from build123d import *

# Parameters (mm, degrees)
F2_DEPTH = 7.62


with BuildPart() as f2:
    # F1 (on Right) → F2 (new body)
    with BuildSketch(Plane.YZ):
        Polygon((-9.930916, 15.784562), (-9.930916, -51.809832), (9.089336, -51.809832), (9.089336, 15.709758), align=None)
        Polygon((-9.930916, -51.809832), (-30.802712, -51.809832), (-30.802712, -67.667425), (48.981383, -67.146659), (48.981383, -51.809832), (9.089336, -51.809832), align=None)
    extrude(amount=-F2_DEPTH)


solid = f2.part
Check sheet for the modelled part. Datum: model origin and axes. Units: mm. A direction names the side the tool comes from. Give positions to 0.01 mm unless a question says otherwise; leave off trailing zeros. Write each loop counter-clockwise with the first axis right and the second up, starting at its lowest first coordinate (ties: lowest second). Pieces come first, ordered by that corner, then holes. Notation, with made-up numbers: (-21, 65) -> (33, 65) arc R20 cw to (33, 72) -> close; hole circle Ø4 at (40, -17.5). An arc over 180 degrees is marked (long way). One line per item, written item: value. Start each with the question number.
Item 1: Material ranges on probe 1 along Y at (x, z) = (-4, -24); probe 2 along Z at (x, y) = (-4.5, 45.5); probe 3 along Z at (x, y) = (-0.75, 8), recorded low to high. Write a range as from..to.
Item 2: Gauge pin test, flat ends, axial feed: pin 1 (3 mm diameter, centred on x = -5, y = 22, fed in from -Z); pin 2 (2.5 mm diameter, centred on x = -2.5, z = -26.5, fed in from -Y); pin 3 (2.5 mm diameter, centred on x = -4.5, y = -16.5, fed in from +Z). Record the tip position at first contact, or that the pin passes through.
Item 3: Tool access check on faces 1 (the flat face through (-4, 29, -51.81)), 2 (the flat face through (-4, -20, -51.81)), 3 (the flat face through (-4, 48.981, -60)). Record the directions out of +Z, -Z, +X, -X, +Y, -Y that give a thin tool (end or side, any length) a straight path to the whole face; none if there is none.
Item 4: Section check B-B on z = -47.5. Record the cut outline in (x, y).
Item 5: Section check C-C on y = -15. Record the cut outline in (x, z), then the cut area to 3 significant figures.
Item 6: Section check A-A on x = -1. Record the cut outline in (y, z), then the cut area to 3 significant figures.
Results list:
1. probe 1: -9.93..9.09
1. probe 2: -67.17..-51.81
1. probe 3: -67.41..15.71
2. pin 1: z = -67.33
2. pin 2: y = -9.93
2. pin 3: z = -51.81
3. face 1: +Z, +X, -X, +Y
3. face 2: +Z, +X, -X, -Y
3. face 3: +Z, -Z, +X, -X, +Y
4. outline: (-7.62, -9.93) -> (0, -9.93) -> (0, 9.09) -> (-7.62, 9.09) -> close
5. outline: (-7.62, -67.56) -> (0, -67.56) -> (0, -51.81) -> (-7.62, -51.81) -> close
5. area: 120 mm²
6. outline: (-30.8, -67.67) -> (48.98, -67.15) -> (48.98, -51.81) -> (9.09, -51.81) -> (9.09, 15.71) -> (-9.93, 15.78) -> (-9.93, -51.81) -> (-30.8, -51.81) -> close
6. area: 2,530 mm²
